```python
from build123d import *

# Parameters (mm, degrees)
SKETCH1_W             = 12
SKETCH1_H             = 58
SKETCH1_R             = 3.25
BOSS_EXTRUDE1_DEPTH   = 4
BOSS_EXTRUDE1_2_DEPTH = 4
BOSS_EXTRUDE2_DEPTH   = 22
SKETCH1_4_W           = 24
SKETCH1_4_H           = 3
BOSS_EXTRUDE3_DEPTH   = 10
SKETCH2_R             = 1.5
BOSS_EXTRUDE4_DEPTH   = 15


with BuildPart() as part:
    # Sketch1 → Boss-Extrude1 (new body)
    with BuildSketch(Plane(origin=(0, 0, 0), x_dir=(1, 0, 0), z_dir=(0, 1, 0))):
        with Locations((-26, 0)):
            Rectangle(SKETCH1_W, SKETCH1_H)
        with Locations((-27, -3)):
            Circle(SKETCH1_R, mode=Mode.SUBTRACT)
    extrude(amount=BOSS_EXTRUDE1_DEPTH)



with BuildPart() as body_2:
    # Sketch1 → Boss-Extrude1 2 (new body)
    with BuildSketch(Plane(origin=(0, 0, 0), x_dir=(1, 0, 0), z_dir=(0, 1, 0))):
        with Locations((26, 0)):
            Rectangle(SKETCH1_W, SKETCH1_H)
        with Locations((27, -3)):
            Circle(SKETCH1_R, mode=Mode.SUBTRACT)
    extrude(amount=BOSS_EXTRUDE1_2_DEPTH)


with BuildPart() as part_1:
    add(part.part)

    add(body_2.part)  # Boss-Extrude2 merges body 2
    # Sketch1<3> → Boss-Extrude2 (add)
    with BuildSketch(Plane(origin=(0, 0, 0), x_dir=(1, 0, 0), z_dir=(0, 1, 0))):
        Polygon((20, 29), (-20, 29), (-20, -29), (-12, -29), (12, -29), (20, -29), align=None)
    extrude(amount=BOSS_EXTRUDE2_DEPTH)

    # Sketch1<4> → Boss-Extrude3 (add)
    with BuildSketch(Plane(origin=(0, 0, 0), x_dir=(1, 0, 0), z_dir=(0, 1, 0))):
        with Locations((0, -30.5)):
            Rectangle(SKETCH1_4_W, SKETCH1_4_H)
    extrude(amount=BOSS_EXTRUDE3_DEPTH)

    # Sketch2 → Boss-Extrude4 (add)
    with BuildSketch(Plane.XY.offset(32)):
        with Locations((-7.5, 3)):
            Circle(SKETCH2_R)
        with Locations((-2.5, 3)):
            Circle(SKETCH2_R)
        with Locations((2.5, 3)):
            Circle(SKETCH2_R)
        with Locations((7.5, 3)):
            Circle(SKETCH2_R)
    extrude(amount=BOSS_EXTRUDE4_DEPTH)


solid = part_1.part
```
Geometry check sheet. Reference: the model listing, model coordinates, mm. A direction names the side the tool comes from. Round coordinates to 2 decimals unless told otherwise and drop trailing zeros. Order: outer loops, then holes, each group sorted by start corner. A loop starts at its lowest first (then second) coordinate and runs counter-clockwise, first axis right, second up. Notation, with made-up numbers: (73.25, 14.5) - (118.25, 14.5) arc R26 cw to (118.25, 42.5) - close; hole circle Ø10 at (-9, 69.5). An arc over 180 degrees is marked (long way). Use a Markdown table: item, result. Add a question column.
(1) Sectioned sample at C-C, the plane y = 3. Enter the section's corners in (x, z), and give its area (3 significant figures).
(2) Release check for a two-part mould opening along X. For faces 1 (the cylindrical face through (-1.81, 1.67, 39.39)), 2 (the flat face through (0, 0, 1)), 3 (the flat face through (32, 2, 0)) record: pulls with the +X half, pulls with the -X half, needs draft (parallel to the pull), parting line crosses it, or undercut.
(3) Tool access check on faces 4 (the flat face through (25.9, 4, -0.4)), 5 (the flat face through (-12, 5, 31)), 6 (the cylindrical face through (6.3, 2.1, 39.4)), 7 (the flat face through (0, 10, 30)), 8 (the flat face through (-20, 13, 0)). Record the directions out of +Z, -Z, +X, -X, +Y, -Y that give a thin tool (end or side, any length) a straight path to the whole face; none if there is none.
(4) Material ranges on line 1 along X through (y, z) = (1.05, 3); line 2 along Z through (x, y) = (27, 1); line 3 along Z through (x, y) = (-15.5, 3), recorded low to high. Write a range as [from, to].
(5) Sectioned sample at B-B, the plane z = 3. Enter the section's corners in (x, y), and give its area (3 significant figures).
(6) Sectioned sample at D-D, the plane x = 7.5. Enter the section's corners in (y, z).
(7) Depth check by flat-ended pin: pin 1 (9 mm diameter, centred on y = 12, z = -5.5, fed in from -X); pin 2 (1.5 mm diameter, centred on y = 6, z = 30.5, fed in from -X); pin 3 (1.5 mm diameter, centred on y = 14.5, z = -20.5, fed in from +X). Enter the tip coordinate at first touch or a pass-through.
(8) Sectioned sample at A-A, the plane x = 27. Enter the section's corners in (y, z).
Answers below:
| question | item | result |
|---|---|---|
| 1 | outline | (-32, -29) - (32, -29) - (32, 29) - (12, 29) - (12, 32) - (9, 32) - (9, 47) - (6, 47) - (6, 32) - (4, 32) - (4, 47) - (1, 47) - (1, 32) - (-1, 32) - (-1, 47) - (-4, 47) - (-4, 32) - (-6, 32) - (-6, 47) - (-9, 47) - (-9, 32) - (-12, 32) - (-12, 29) - (-32, 29) - close; hole circle Ø6.5 at (-27, 3); hole circle Ø6.5 at (27, 3) |
| 1 | area | 3,900 mm² |
| 2 | face 1 | undercut |
| 2 | face 2 | needs draft |
| 2 | face 3 | pulls with the +X half |
| 3 | face 4 | +Z, -Z, +X, +Y |
| 3 | face 5 | +Z, -X, +Y, -Y |
| 3 | face 6 | +Z |
| 3 | face 7 | +Z, +X, -X, +Y |
| 3 | face 8 | +Z, -Z, -X, +Y |
| 4 | line 1 | [-32, -30.25], [-23.75, 23.75], [30.25, 32] |
| 4 | line 2 | [-29, -0.25], [6.25, 29] |
| 4 | line 3 | [-29, 29] |
| 5 | outline | (-32, 0) - (-30.25, 0) - (-30.25, 4) - (-32, 4) - close; (-23.75, 0) - (23.75, 0) - (23.75, 4) - (20, 4) - (20, 22) - (-20, 22) - (-20, 4) - (-23.75, 4) - close; (30.25, 0) - (32, 0) - (32, 4) - (30.25, 4) - close |
| 5 | area | 924 mm² |
| 6 | outline | (0, -29) - (22, -29) - (22, 29) - (10, 29) - (10, 32) - (4.5, 32) - (4.5, 47) - (1.5, 47) - (1.5, 32) - (0, 32) - close |
| 7 | pin 1 | x = -20 |
| 7 | pin 2 | x = -12 |
| 7 | pin 3 | x = 20 |
| 8 | outline | (0, -29) - (4, -29) - (4, -0.25) - (0, -0.25) - close; (0, 6.25) - (4, 6.25) - (4, 29) - (0, 29) - close |
